from build123d import *

# Parameters (mm, degrees)
F0_W     = 88.9
F0_H     = 25.4
F1_DEPTH = 3.175
F2_W     = 88.9
F2_H     = 3.175
F3_DEPTH = 12.7
F5_D     = 3.3
F7_DEPTH = 3.175
F8_R     = 3.175


with BuildPart() as f1:
    # F0 (on Top) → F1 (new body)
    with BuildSketch(Plane.XY):
        Rectangle(F0_W, F0_H)
    extrude(amount=F1_DEPTH)

    # F2 (on face) → F3 (join)
    with BuildSketch(Plane(origin=(0, 0, 0), x_dir=(1, 0, 0), z_dir=(0, 0, -1))):
        with Locations((0, 11.1125)):
            Rectangle(F2_W, F2_H)
        with Locations((0, -11.1125)):
            Rectangle(F2_W, F2_H)
    extrude(amount=F3_DEPTH)

    # F5 (through all)
    with Locations(Plane.XY.offset(3.175)):
        with Locations((-38.89375, 0), (38.89375, 0)):
            Hole(F5_D / 2)

    # F6 (on face) → F7 (cut)
    with BuildSketch(Plane.XZ.offset(12.7)):
        with BuildLine():
            Line((-31.353125, -8.636), (-24.209375, -8.636))
            ThreePointArc((-24.209375, -8.636), (-27.78125, -5.064125), (-31.353125, -8.636))
        make_face()
        with BuildLine():
            Line((-24.209375, -12.7), (-24.209375, -8.636))
            ThreePointArc((-24.209375, -8.636), (-27.78125, -12.207875), (-31.353125, -8.636))
            Line((-31.353125, -8.636), (-31.353125, -12.7))
            Line((-31.353125, -12.7), (-24.209375, -12.7))
        make_face()
        with BuildLine():
            ThreePointArc((-31.353125, -8.636), (-27.78125, -12.207875), (-24.209375, -8.636))
            Line((-24.209375, -8.636), (-31.353125, -8.636))
        make_face()
        with BuildLine():
            Line((-20.240625, -8.636), (-13.096875, -8.636))
            ThreePointArc((-13.096875, -8.636), (-16.66875, -5.064125), (-20.240625, -8.636))
        make_face()
        with BuildLine():
            Line((-13.096875, -12.7), (-13.096875, -8.636))
            ThreePointArc((-13.096875, -8.636), (-16.66875, -12.207875), (-20.240625, -8.636))
            Line((-20.240625, -8.636), (-20.240625, -12.7))
            Line((-20.240625, -12.7), (-13.096875, -12.7))
        make_face()
        with BuildLine():
            ThreePointArc((-20.240625, -8.636), (-16.66875, -12.207875), (-13.096875, -8.636))
            Line((-13.096875, -8.636), (-20.240625, -8.636))
        make_face()
        with BuildLine():
            Line((-9.128125, -8.636), (-1.984375, -8.636))
            ThreePointArc((-1.984375, -8.636), (-5.55625, -5.064125), (-9.128125, -8.636))
        make_face()
        with BuildLine():
            Line((-1.984375, -12.7), (-1.984375, -8.636))
            ThreePointArc((-1.984375, -8.636), (-5.55625, -12.207875), (-9.128125, -8.636))
            Line((-9.128125, -8.636), (-9.128125, -12.7))
            Line((-9.128125, -12.7), (-1.984375, -12.7))
        make_face()
        with BuildLine():
            ThreePointArc((-9.128125, -8.636), (-5.55625, -12.207875), (-1.984375, -8.636))
            Line((-1.984375, -8.636), (-9.128125, -8.636))
        make_face()
        with BuildLine():
            Line((1.984375, -8.636), (9.128125, -8.636))
            ThreePointArc((9.128125, -8.636), (5.55625, -5.064125), (1.984375, -8.636))
        make_face()
        with BuildLine():
            Line((9.128125, -12.7), (9.128125, -8.636))
            ThreePointArc((9.128125, -8.636), (5.55625, -12.207875), (1.984375, -8.636))
            Line((1.984375, -8.636), (1.984375, -12.7))
            Line((1.984375, -12.7), (9.128125, -12.7))
        make_face()
        with BuildLine():
            ThreePointArc((1.984375, -8.636), (5.55625, -12.207875), (9.128125, -8.636))
            Line((9.128125, -8.636), (1.984375, -8.636))
        make_face()
        with BuildLine():
            Line((13.096875, -8.636), (20.240625, -8.636))
            ThreePointArc((20.240625, -8.636), (16.66875, -5.064125), (13.096875, -8.636))
        make_face()
        with BuildLine():
            Line((20.240625, -12.7), (20.240625, -8.636))
            ThreePointArc((20.240625, -8.636), (16.66875, -12.207875), (13.096875, -8.636))
            Line((13.096875, -8.636), (13.096875, -12.7))
            Line((13.096875, -12.7), (20.240625, -12.7))
        make_face()
        with BuildLine():
            ThreePointArc((13.096875, -8.636), (16.66875, -12.207875), (20.240625, -8.636))
            Line((20.240625, -8.636), (13.096875, -8.636))
        make_face()
        with BuildLine():
            Line((24.209375, -8.636), (31.353125, -8.636))
            ThreePointArc((31.353125, -8.636), (27.78125, -5.064125), (24.209375, -8.636))
        make_face()
        with BuildLine():
            Line((31.353125, -12.7), (31.353125, -8.636))
            ThreePointArc((31.353125, -8.636), (27.78125, -12.207875), (24.209375, -8.636))
            Line((24.209375, -8.636), (24.209375, -12.7))
            Line((24.209375, -12.7), (31.353125, -12.7))
        make_face()
        with BuildLine():
            ThreePointArc((24.209375, -8.636), (27.78125, -12.207875), (31.353125, -8.636))
            Line((31.353125, -8.636), (24.209375, -8.636))
        make_face()
    extrude(amount=-F7_DEPTH, mode=Mode.SUBTRACT)

    # F8
    f8_edges = [f1.edges().sort_by_distance(p)[0] for p in [
        (0, -12.7, 3.175),
        (0, 12.7, 3.175),
    ]]
    fillet(f8_edges, radius=F8_R)


solid = f1.part
The model under review builds one solid part; all positions refer to its coordinate system, in mm. A direction names the side the tool comes from. Give positions to 0.01 mm unless a question says otherwise; leave off trailing zeros. Order: outer loops, then holes, each group sorted by start corner. A loop starts at its lowest first (then second) coordinate and runs counter-clockwise, first axis right, second up. Notation, with made-up numbers: M -38.5,62.5 L 10.5,62.5 A11 cw 10.5,81.5 Z; hole C 33,8 d3. An arc over 180 degrees is marked long. Use one line per item in the form item = value. Start each with the question number.
Item 1: We need section B-B on z = -1.5. Give the boundary of the cut face in (x, y) (3 decimals), plus the area to 3 significant figures.
Item 2: To check wall thickness, follow line 1 along Y through (x, z) = (-15.5, -4.25) (3 decimals); line 2 along Z through (x, y) = (-20, -1) (3 decimals); line 3 along Y through (x, z) = (3, -9) (3 decimals). State the ranges of each line that lie inside material, in increasing order. Write a range as from..to.
Item 3: We need section C-C on z = -10.75. Give the number of separate pieces and of enclosed holes in the cut face, plus the area to 3 significant figures.
Item 4: Insertion check: pin 1 Ø4 at (x, y) = (3.5, -6) entering from -Z. The pin has a flat end and moves straight along its axis. Give the tip position at first contact, or say it passes through.
Item 5: The part is to be moulded in two halves that separate along X. For faces 1 (the cylindrical face through (40.542, 0.073, 1.565)), 2 (the flat face through (-11, -11, -12.7)), 3 (the flat face through (-44.45, 0, 1)), 4 (the flat face through (-13.097, -11, -11)), say which applies: pulls with the +X half, pulls with the -X half, needs draft (parallel to the pull), parting line crosses it, or undercut.
Item 6: For faces 5 (the flat face through (-1, -12.7, -6)), 6 (the cylindrical face through (27.86, -11.135, -5.065)), 7 (the flat face through (-1, -9.525, -6)), list the 3-axis set-ups (+Z, -Z, +X, -X, +Y, -Y) from which the entire face can be reached by the end or side of a thin tool; tool diameter is ignored.
Item 7: We need section A-A on y = 0. Give the boundary of the cut face in (x, z) (3 decimals).
Item 8: We need section D-D on x = -10. Give the boundary of the cut face in (y, z) (3 decimals).
Completed:
q1.outline = M -44.45,-12.7 L 44.45,-12.7 L 44.45,-9.525 L -44.45,-9.525 Z; M -44.45,9.525 L 44.45,9.525 L 44.45,12.7 L -44.45,12.7 Z
q1.area = 565 mm²
q2.line_1 = -12.7..-9.525, 9.525..12.7
q2.line_2 = 0..3.175
q2.line_3 = 9.525..12.7
q3.separate_pieces = 8
q3.enclosed_holes = 0
q3.area = 428 mm²
q4.pin_1 = 0
q5.face_1 = undercut
q5.face_2 = needs draft
q5.face_3 = pulls with the -X half
q5.face_4 = undercut
q6.face_5 = +Z, -Z, +X, -X, -Y
q6.face_6 = -Z, -Y
q6.face_7 = -Z, +X, -X
q7.outline = M -44.45,0 L -40.544,0 L -40.544,3.175 L -44.45,3.175 Z; M -37.244,0 L 37.244,0 L 37.244,3.175 L -37.244,3.175 Z; M 40.544,0 L 44.45,0 L 44.45,3.175 L 40.544,3.175 Z
q8.outline = M -12.7,-12.7 L -9.525,-12.7 L -9.525,0 L 9.525,0 L 9.525,-12.7 L 12.7,-12.7 L 12.7,0 A3.175 ccw 9.525,3.175 L -9.525,3.175 A3.175 ccw -12.7,0 Z
